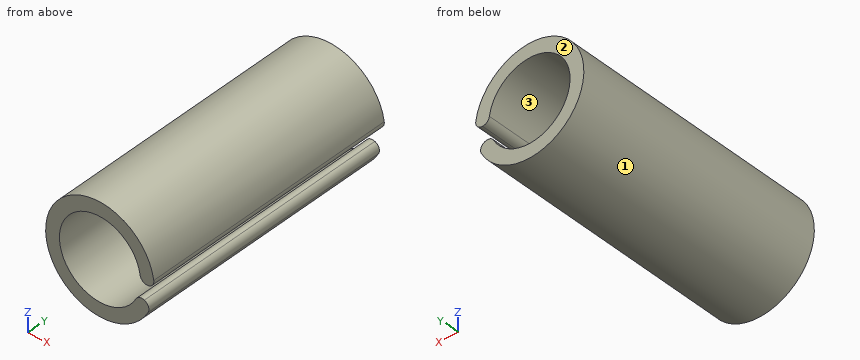
from build123d import *

# Parameters (mm, degrees)
BOSS_EXTRUDE1_DEPTH = 15
FILLET1_R           = 0.4


with BuildPart() as part:
    # Sketch1 → Boss-Extrude1 (new body)
    with BuildSketch(Plane(origin=(0, 0, 0), x_dir=(1, 0, 0), z_dir=(0, 1, 0))):
        with BuildLine():
            Line((2.219557977, 0.772050767), (2.971014846, 1.046695174))
            ThreePointArc((2.971014846, 1.046695174), (-3.104931301, -0.530944082), (3.15, 0))
            Line((3.15, 0), (2.35, 0))
            ThreePointArc((2.35, 0), (-2.317160034, -0.391496331), (2.219557977, 0.772050767))
        make_face()
    extrude(amount=BOSS_EXTRUDE1_DEPTH)

    # Fillet1
    fillet1_edges = [part.edges().sort_by_distance(p)[0] for p in [
        (3.15, 7.5, 0),
        (2.35, 7.5, 0),
        (2.219557977, 7.5, -0.772050767),
        (2.971014846, 7.5, -1.046695174),
    ]]
    fillet(fillet1_edges, radius=FILLET1_R - 0.0001)  # a hair under: the kernel refuses the full size


solid = part.part
Source: CAD feature listing. Evaluate the final solid. Frame: model axes, mm. Face numbers are marked on the shaded views. Give positions to 0.01 mm unless a question says otherwise; leave off trailing zeros. Loops run counter-clockwise (first coordinate to the right, second up) from the corner with the lowest first, then second, coordinate; pieces in that order, holes last. Notation, with made-up numbers: (21, 62.5) -> (55, 62.5) arc R29 ccw to (55, 91.5) -> close; hole circle Ø9 at (67, 47.5). An arc over 180 degrees is marked (long way). Use a Markdown table: item, result. Add a question column.
1) Section query C-C, the plane x = -1. Return the cut outline in (y, z).
2) Section query D-D, the plane z = 2.5. Return the cut outline in (x, y).
3) Line query: line 1 along Z through (x, y) = (0, 3.25); line 2 along X through (y, z) = (3.5, -2); line 3 along Z through (x, y) = (1.5, 8). Output: solid intervals per line, ascending. Write a range as [from, to].
4) Section query A-A, the plane x = 0. Return the cut outline in (y, z).
5) First-contact query: pin 1 (1.5 mm diameter, centred on x = 2, y = 2.5, fed in from -Z). Flat tip, straight axial feed; report the tip coordinate or a pass-through.
6) Pull-direction query (Z, two-part tool) for the marked faces 1, 2 and 3; classes: +Z half, -Z half, draft (parallel to the pull), parting line (faces both ways), or undercut.
Numbers:
| question | item | result |
|---|---|---|
| 1 | outline | (0, -2.99) -> (15, -2.99) -> (15, -2.13) -> (0, -2.13) -> close; (0, 2.13) -> (15, 2.13) -> (15, 2.99) -> (0, 2.99) -> close |
| 2 | outline | (-1.92, 0) -> (1.92, 0) -> (1.92, 15) -> (-1.92, 15) -> close |
| 3 | line 1 | z = [-3.15, -2.35], [2.35, 3.15] |
| 3 | line 2 | x = [-2.43, -1.23], [1.23, 2.43] |
| 3 | line 3 | z = [-2.77, -1.81], [1.81, 2.77] |
| 4 | outline | (0, -3.15) -> (15, -3.15) -> (15, -2.35) -> (0, -2.35) -> close; (0, 2.35) -> (15, 2.35) -> (15, 3.15) -> (0, 3.15) -> close |
| 5 | pin 1 | stops at z = -2.89 |
| 6 | face 1 | parting line |
| 6 | face 2 | draft |
| 6 | face 3 | undercut |
